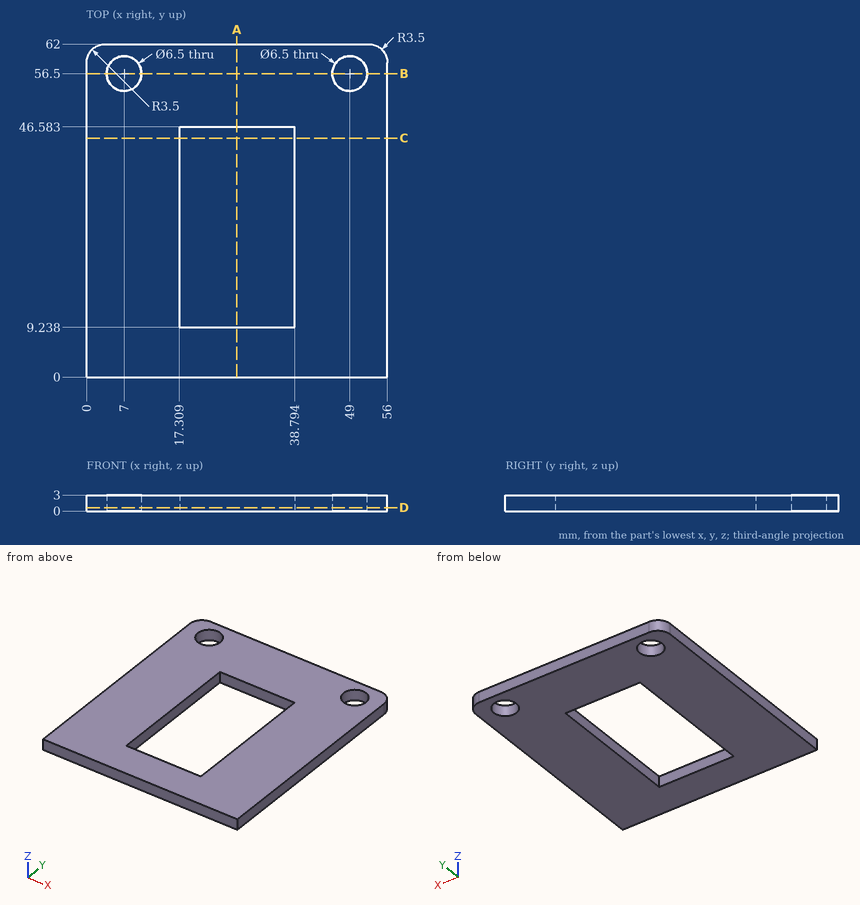
Input: dimensioned drawing with shaded views. Units: mm. Origin: part minimum x, y, z. Coordinates: 2 decimals unless noted, no trailing zeros. Order: outer loops, then holes, each group sorted by start corner. A loop starts at its lowest first (then second) coordinate and runs counter-clockwise, first axis right, second up.
(1) Section query B-B (y = 56.5). Return the cut outline in (x, z).
(2) Section query C-C (y = 44.5). Return the cut outline in (x, z).
(3) Section query D-D (z = 0.65). Return the cut outline in (x, y), plus the area to 3 significant figures.
(4) Section query A-A (x = 28). Return the cut outline in (y, z).
(5) Material intervals for probe 1 along X at (y, z) = (56.5, 1.6); probe 2 along Y at (x, z) = (49, 2.2); probe 3 along X at (y, z) = (13.5, 0.2), sorted ascending.
Solution:
1. outline: (0, 0) - (3.75, 0) - (3.75, 3) - (0, 3) - close; (10.25, 0) - (45.75, 0) - (45.75, 3) - (10.25, 3) - close; (52.25, 0) - (56, 0) - (56, 3) - (52.25, 3) - close
2. outline: (0, 0) - (17.31, 0) - (17.31, 3) - (0, 3) - close; (38.79, 0) - (56, 0) - (56, 3) - (38.79, 3) - close
3. outline: (0, 0) - (56, 0) - (56, 58.5) arc R3.5 ccw to (52.5, 62) - (3.5, 62) arc R3.5 ccw to (0, 58.5) - close; hole circle Ø6.5 at (7, 56.5); hole (17.31, 9.24) - (38.79, 9.24) - (38.79, 46.58) - (17.31, 46.58) - close; hole circle Ø6.5 at (49, 56.5)
3. area: 2,600 mm2
4. outline: (0, 0) - (9.24, 0) - (9.24, 3) - (0, 3) - close; (46.58, 0) - (62, 0) - (62, 3) - (46.58, 3) - close
5. probe 1: x = 0 to 3.75, 10.25 to 45.75, 52.25 to 56
5. probe 2: y = 0 to 53.25, 59.75 to 62
5. probe 3: x = 0 to 17.31, 38.79 to 56
